Geometry: final body of the model. Coordinates: model frame, mm. Give positions to 0.01 mm unless a question says otherwise; leave off trailing zeros. Loops run counter-clockwise (first coordinate to the right, second up) from the corner with the lowest first, then second, coordinate; pieces in that order, holes last. Notation, with made-up numbers: M -28,47.25 L 31,47.25 A24 cw 31,67.25 Z; hole C 23.25,75 d10. An arc over 180 degrees is marked long. Put each result on its own line as item: value.
```python
from build123d import *

# Parameters (mm, degrees)
SKETCH1_R           = 9
BOSS_EXTRUDE1_DEPTH = 4


with BuildPart() as part:
    # Sketch1 → Boss-Extrude1 (new body)
    with BuildSketch(Plane.XY):
        with BuildLine():
            ThreePointArc((3.504747833, 20.671687749), (2.214882396, 19.700607102), (1.173151508, 20.934117224))
            ThreePointArc((1.173151508, 20.934117224), (1.173961835, 20.950617719), (1.174540093, 20.967127976))
            ThreePointArc((1.174540093, 20.967127976), (0, 22.175), (-1.174540093, 20.967127976))
            ThreePointArc((-1.174540093, 20.967127976), (-1.173961835, 20.950617719), (-1.173151508, 20.934117224))
            ThreePointArc((-1.173151508, 20.934117224), (-2.214882396, 19.700607102), (-3.504747833, 20.671687749))
            ThreePointArc((-3.504747833, 20.671687749), (-4.924249618, 21.620773739), (-5.792423756, 20.150391748))
            ThreePointArc((-5.792423756, 20.150391748), (-6.534230721, 18.716350991), (-8.007531076, 19.376757329))
            ThreePointArc((-8.007531076, 19.376757329), (-9.602346953, 19.986930953), (-10.122330354, 18.360472593))
            ThreePointArc((-10.122330354, 18.360472593), (-10.527171603, 16.797509372), (-12.110338295, 17.114264311))
            ThreePointArc((-12.110338295, 17.114264311), (-13.800831861, 17.355056827), (-13.94665939, 15.653738554))
            ThreePointArc((-13.94665939, 15.653738554), (-13.994319359, 14.039898725), (-15.608297681, 13.997185253))
            ThreePointArc((-15.608297681, 13.997185253), (-17.310054912, 13.856572796), (-17.074444737, 12.165349162))
            ThreePointArc((-17.074444737, 12.165349162), (-16.762543548, 10.581219081), (-18.32674023, 10.181170075))
            ThreePointArc((-18.32674023, 10.181170075), (-19.954784653, 9.666174064), (-19.349501862, 8.06949555))
            ThreePointArc((-19.349501862, 8.06949555), (-18.693614158, 6.59417803), (-20.129921751, 5.856769754))
            ThreePointArc((-20.129921751, 5.856769754), (-21.602957711, 4.993106281), (-20.658226823, 3.570702301))
            ThreePointArc((-20.658226823, 3.570702301), (-19.691104059, 2.277866648), (-20.927801198, 1.23992125))
            ThreePointArc((-20.927801198, 1.23992125), (-20.94927463, 1.240996152), (-20.970764135, 1.241677968))
            ThreePointArc((-20.970764135, 1.241677968), (-22.172279268, 0.066977177), (-20.970764135, -1.107723614))
            ThreePointArc((-20.970764135, -1.107723614), (-20.94927463, -1.107041799), (-20.927801198, -1.105966896))
            ThreePointArc((-20.927801198, -1.105966896), (-19.691104059, -2.143912295), (-20.658226823, -3.436747947))
            ThreePointArc((-20.658226823, -3.436747947), (-21.602957711, -4.859151928), (-20.129921751, -5.722815401))
            ThreePointArc((-20.129921751, -5.722815401), (-18.693614158, -6.460223676), (-19.349501862, -7.935541197))
            ThreePointArc((-19.349501862, -7.935541197), (-19.954784653, -9.532219711), (-18.32674023, -10.047215721))
            ThreePointArc((-18.32674023, -10.047215721), (-16.762543548, -10.447264727), (-17.074444737, -12.031394809))
            ThreePointArc((-17.074444737, -12.031394809), (-17.310054912, -13.722618442), (-15.608297681, -13.863230899))
            ThreePointArc((-15.608297681, -13.863230899), (-13.994319359, -13.905944371), (-13.94665939, -15.5197842))
            ThreePointArc((-13.94665939, -15.5197842), (-13.800831861, -17.221102473), (-12.110338295, -16.980309958))
            ThreePointArc((-12.110338295, -16.980309958), (-10.527171603, -16.663555018), (-10.122330354, -18.226518239))
            ThreePointArc((-10.122330354, -18.226518239), (-9.602346953, -19.852976599), (-8.007531076, -19.242802976))
            ThreePointArc((-8.007531076, -19.242802976), (-6.534230721, -18.582396638), (-5.792423756, -20.016437395))
            ThreePointArc((-5.792423756, -20.016437395), (-4.924249618, -21.486819385), (-3.504747833, -20.537733396))
            ThreePointArc((-3.504747833, -20.537733396), (-2.214882396, -19.566652749), (-1.173151508, -20.800162871))
            ThreePointArc((-1.173151508, -20.800162871), (-1.173961835, -20.816663366), (-1.174540093, -20.833173623))
            ThreePointArc((-1.174540093, -20.833173623), (0, -22.041045646), (1.174540093, -20.833173623))
            ThreePointArc((1.174540093, -20.833173623), (1.173961835, -20.816663366), (1.173151508, -20.800162871))
            ThreePointArc((1.173151508, -20.800162871), (2.214882396, -19.566652749), (3.504747833, -20.537733396))
            ThreePointArc((3.504747833, -20.537733396), (4.924249618, -21.486819385), (5.792423756, -20.016437395))
            ThreePointArc((5.792423756, -20.016437395), (6.534230721, -18.582396638), (8.007531076, -19.242802976))
            ThreePointArc((8.007531076, -19.242802976), (9.602346953, -19.852976599), (10.122330354, -18.226518239))
            ThreePointArc((10.122330354, -18.226518239), (10.527171603, -16.663555018), (12.110338295, -16.980309958))
            ThreePointArc((12.110338295, -16.980309958), (13.800831861, -17.221102473), (13.94665939, -15.5197842))
            ThreePointArc((13.94665939, -15.5197842), (13.994319359, -13.905944371), (15.608297681, -13.863230899))
            ThreePointArc((15.608297681, -13.863230899), (17.310054912, -13.722618442), (17.074444737, -12.031394809))
            ThreePointArc((17.074444737, -12.031394809), (16.762543548, -10.447264727), (18.32674023, -10.047215721))
            ThreePointArc((18.32674023, -10.047215721), (19.954784653, -9.532219711), (19.349501862, -7.935541197))
            ThreePointArc((19.349501862, -7.935541197), (18.693614158, -6.460223676), (20.129921751, -5.722815401))
            ThreePointArc((20.129921751, -5.722815401), (21.602957711, -4.859151928), (20.658226823, -3.436747947))
            ThreePointArc((20.658226823, -3.436747947), (19.691104059, -2.143912295), (20.927801198, -1.105966896))
            ThreePointArc((20.927801198, -1.105966896), (20.94927463, -1.107041799), (20.970764135, -1.107723614))
            ThreePointArc((20.970764135, -1.107723614), (22.172279268, 0.066977177), (20.970764135, 1.241677968))
            ThreePointArc((20.970764135, 1.241677968), (20.94927463, 1.240996152), (20.927801198, 1.23992125))
            ThreePointArc((20.927801198, 1.23992125), (19.691104059, 2.277866648), (20.658226823, 3.570702301))
            ThreePointArc((20.658226823, 3.570702301), (21.602957711, 4.993106281), (20.129921751, 5.856769754))
            ThreePointArc((20.129921751, 5.856769754), (18.693614158, 6.59417803), (19.349501862, 8.06949555))
            ThreePointArc((19.349501862, 8.06949555), (19.954784653, 9.666174064), (18.32674023, 10.181170075))
            ThreePointArc((18.32674023, 10.181170075), (16.762543548, 10.581219081), (17.074444737, 12.165349162))
            ThreePointArc((17.074444737, 12.165349162), (17.310054912, 13.856572796), (15.608297681, 13.997185253))
            ThreePointArc((15.608297681, 13.997185253), (13.994319359, 14.039898725), (13.94665939, 15.653738554))
            ThreePointArc((13.94665939, 15.653738554), (13.800831861, 17.355056827), (12.110338295, 17.114264311))
            ThreePointArc((12.110338295, 17.114264311), (10.527171603, 16.797509372), (10.122330354, 18.360472593))
            ThreePointArc((10.122330354, 18.360472593), (9.602346953, 19.986930953), (8.007531076, 19.376757329))
            ThreePointArc((8.007531076, 19.376757329), (6.534230721, 18.716350991), (5.792423756, 20.150391748))
            ThreePointArc((5.792423756, 20.150391748), (4.924249618, 21.620773739), (3.504747833, 20.671687749))
        make_face()
        Circle(SKETCH1_R, mode=Mode.SUBTRACT)
    extrude(amount=BOSS_EXTRUDE1_DEPTH)


solid = part.part
```
Item 1: Pin query (flat end, axial travel): pin 1 Ø2 at (x, y) = (-16, 5) entering from -Z; pin 2 Ø2 at (y, z) = (-15, 2.5) entering from +X; pin 3 Ø1.5 at (x, z) = (-6, 3) entering from +Y. Return the tip coordinate at first contact, or that it passes through.
Output values:
pin 1: z = 0
pin 2: x = 16.99
pin 3: y = 21.49
Item 2: Mould query, pull axis Y, two halves, no side actions, for faces 1 (the flat face through (-0.3, -9.4, 0)), 2 (the cylindrical face through (-1.172, 8.923, 1.972)). Classes: pulls with the +Y half, pulls with the -Y half, needs draft (parallel to the pull), parting line crosses it, or undercut.
Output values:
face 1: needs draft
face 2: undercut
Item 3: Section B-B on y = 0. Output: boundary loops of the cut face in (x, z).
Output values:
outline: M -22.17,0 L -9,0 L -9,4 L -22.17,4 Z; M 9,0 L 22.17,0 L 22.17,4 L 9,4 Z
Item 4: Line query: probe 1 along Y at (x, z) = (20.5, 2.85); probe 2 along Y at (x, z) = (0, 2.25) (3 decimals); probe 3 along Y at (x, z) = (-11, 1.6). Output: solid intervals per line, ascending. Write a range as [from, to].
Output values:
probe 1: [-5.77, -3.4], [-1.16, 1.29], [3.53, 5.9]
probe 2: [-22.041, -9], [9, 22.175]
probe 3: [-16.49, 16.63]
Item 5: Section A-A on x = 0. Output: boundary loops of the cut face in (y, z) (3 decimals).
Output values:
outline: M -22.041,0 L -9,0 L -9,4 L -22.041,4 Z; M 9,0 L 22.175,0 L 22.175,4 L 9,4 Z
